from build123d import *

# Parameters (mm, degrees)
FILLET1_R = 1.27


with BuildPart() as part:
    # Sketch1 → Revolve1 (revolve)
    with BuildSketch(Plane.XY, mode=Mode.PRIVATE) as revolve1_sk:
        Polygon((13.081, 0), (14.351, 0), (14.351, 12.7), (6.35, 12.7), (2.54, 45.212), (1.410137462, 45.212), (1.410137462, 43.942), (5.220137462, 11.43), (13.081, 11.43), (13.081, 1.27), align=None)
    revolve(revolve1_sk.sketch.rotate(Axis((0, 43.942, 0), (0, -1, 0)), 180), axis=Axis((0, 43.942, 0), (0, -1, 0)))

    # Fillet1
    fillet1_edges = [part.edges().sort_by_distance(p)[0] for p in [
        (2.54, 45.212, 0),
        (6.35, 12.7, 0),
        (14.351, 12.7, 0),
        (14.351, 0, 0),
    ]]
    fillet(fillet1_edges, radius=FILLET1_R - 0.0001)  # a hair under: the kernel refuses the full size


solid = part.part
Geometry: final body of the model. Coordinates: model frame, mm. A direction names the side the tool comes from. Round coordinates to 2 decimals unless told otherwise and drop trailing zeros. Loops run counter-clockwise (first coordinate to the right, second up) from the corner with the lowest first, then second, coordinate; pieces in that order, holes last. Notation, with made-up numbers: (35, 68.25) - (69, 68.25) arc R17 cw to (69, 76.25) - close; hole circle Ø10 at (43, 70.25). An arc over 180 degrees is marked (long way). Write each question's results on one line, items separated by ' | '. Start each with the question number.
1) Mould query, pull axis Z, two halves, no side actions, for faces 1 (the face through (6, 11.43, 0)), 2 (the face through (1, 29.2, 4.3)), 3 (the face through (-6, 12.7, 6)). Classes: released by +Z, released by -Z, zero draft, split by the parting line, or undercut.
2) Access query for faces 4 (the face through (2.84, 5.63, 12.77)), 5 (the face through (0.306, 44.568, 1.377)). Directions: +Z, -Z, +X, -X, +Y, -Y. A direction counts if a zero-diameter tool reaches every point of the face in a straight line with its end or side. Return the directions, or none.
3) Cut plane C-C on y = 7. Return loops of the section in (x, z), then the cut area to 3 significant figures.
4) Cut plane D-D on y = 40. Return loops of the section in (x, z), then the cut area to 3 significant figures.
5) Line query: probe 1 along Z at (x, y) = (0, 6); probe 2 along Y at (x, z) = (-2.25, 8.75); probe 3 along Y at (x, z) = (10.75, -7.5). Output: solid intervals per line, ascending. Write a range as [from, to].
6) First-contact query: P1, Ø5, axis at y = 13.5, z = 4, coming from the +X side; P2, Ø5, axis at x = 4.5, z = 9, coming from the -Y side; P3, Ø8, axis at y = 22.5, z = 8, coming from the -X side. Flat tips, straight axial feed; report the tip coordinate or a pass-through.
Verdict:
1) face 1: undercut | face 2: split by the parting line | face 3: zero draft
2) face 4: -Y | face 5: +Y, -Y
3) outline: circle Ø28.7 at (0, 0); hole circle Ø26.16 at (0, 0) | area: 109 mm2
4) outline: circle Ø6.3 at (0, 0); hole circle Ø3.74 at (0, 0) | area: 20.2 mm2
5) probe 1: z = [-14.35, -13.08], [13.08, 14.35] | probe 2: y = [11.43, 12.7] | probe 3: y = [0, 12.7]
6) P1: stops at x = 14.14 | P2: stops at y = 11.43 | P3: stops at x = -3.38
